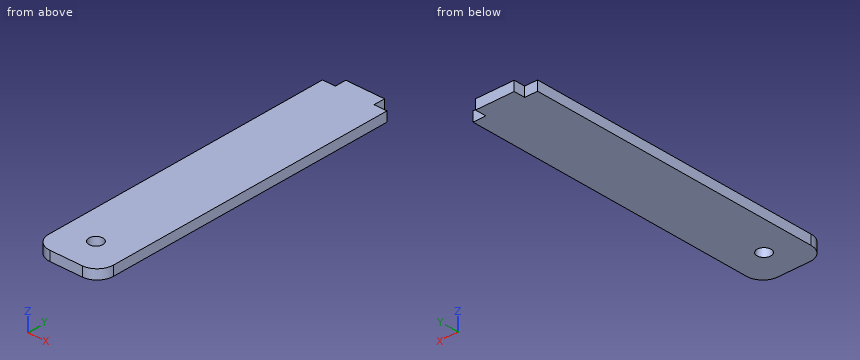
from build123d import *

# Parameters (mm, degrees)
SKETCH_1_R      = 2.15
EXTRUDE_1_DEPTH = 3
FILLET_1_R      = 5


with BuildPart() as part:
    # 草图1 → 凸台-拉伸1 (new body)
    with BuildSketch(Plane.XY):
        Polygon((16, 97), (20, 97), (20, 0), (0, 0), (0, 97), (4, 97), (4, 100.5), (16, 100.5), align=None)
        with Locations((10, 10)):
            Circle(SKETCH_1_R, mode=Mode.SUBTRACT)
    extrude(amount=EXTRUDE_1_DEPTH)

    # 圆角1
    fillet_1_edges = [part.edges().sort_by_distance(p)[0] for p in [
        (20, 0, 1.5),
        (0, 0, 1.5),
    ]]
    fillet(fillet_1_edges, radius=FILLET_1_R)


solid = part.part
The listing builds one solid part. Answer for the finished solid, in the listing's coordinates (mm). Give positions to 0.01 mm unless a question says otherwise; leave off trailing zeros. Write each loop counter-clockwise with the first axis right and the second up, starting at its lowest first coordinate (ties: lowest second). Pieces come first, ordered by that corner, then holes.
1) Section B-B (x = 10) is taken. Write down the section's boundary in (y, z).
2) Find the intervals of material crossed by L1, parallel to Y at x = 10, z = 2.1; L2, parallel to Y at x = 9, z = 2.1; L3, parallel to Y at x = 4.75, z = 1.8, in increasing order.
3) Section C-C (y = 10) is taken. Write down the section's boundary in (x, z).
4) Section D-D (x = 2.5) is taken. Write down the section's boundary in (y, z).
5) Section A-A (z = 0.8) is taken. Write down the section's boundary in (x, y), and give its area (3 significant figures).
6) Given P1, Ø1.5, axis at x = 18, z = 1.5, coming from the +Y side, flat-ended and moving along its own axis, determine where the tip first touches the part or whether it passes through.
Response:
1. outline: (0, 0) - (7.85, 0) - (7.85, 3) - (0, 3) - close; (12.15, 0) - (100.5, 0) - (100.5, 3) - (12.15, 3) - close
2. L1: y = 0 to 7.85, 12.15 to 100.5
2. L2: y = 0 to 8.1, 11.9 to 100.5
2. L3: y = 0.01 to 100.5
3. outline: (0, 0) - (7.85, 0) - (7.85, 3) - (0, 3) - close; (12.15, 0) - (20, 0) - (20, 3) - (12.15, 3) - close
4. outline: (0.67, 0) - (97, 0) - (97, 3) - (0.67, 3) - close
5. outline: (0, 5) arc R5 ccw to (5, 0) - (15, 0) arc R5 ccw to (20, 5) - (20, 97) - (16, 97) - (16, 100.5) - (4, 100.5) - (4, 97) - (0, 97) - close; hole circle Ø4.3 at (10, 10)
5. area: 1,960 mm2
6. P1: stops at y = 97
